Can you work these out from the model? Positions are in its coordinate system, mm. Face numbers are marked on the shaded views. A direction names the side the tool comes from. Coordinates: 2 decimals unless noted, no trailing zeros. Order: outer loops, then holes, each group sorted by start corner. A loop starts at its lowest first (then second) coordinate and runs counter-clockwise, first axis right, second up. Notation, with made-up numbers: (20.5, 68) -> (67.5, 68) arc R16 ccw to (67.5, 83) -> close; hole circle Ø9 at (9, -23). An arc over 180 degrees is marked (long way). Return JSON: item names as keys, results as strings. Group by question number.
1) If we section it at C-C, the plane y = 11: Please give me the cut outline in (x, z) (3 decimals).
2) Thinking about a two-plate mould opening in Y: for the marked faces 3, 4 and 5, which applies, +Y half, -Y half, draft (parallel to the pull), parting line (faces both ways), or undercut?
3) For the marked faces 1 and 2, which set-ups out of +Z, -Z, +X, -X, +Y, -Y let a thin tool reach every point of the face, with its end or its side?
4) For pin 1 (3 mm diameter, centred on x = 8.5, y = 8.5, fed in from -Z); pin 2 (1 mm diameter, centred on x = 4, y = 11.5, fed in from +Z); pin 3 (10 mm diameter, centred on x = -10, z = 3, fed in from -Y); pin 4 (3 mm diameter, centred on y = 2.5, z = 7.5, fed in from +X), each with a flat end and sliding along its axis, tell me the tip position at first contact or that it passes through.
5) If I drill on probe 1 along Z at (x, y) = (0, 9.5) (3 decimals); probe 2 along Z at (x, y) = (0, 3.75); probe 3 along Y at (x, z) = (7.5, 7.5), over which ranges is the centre line in solid material (lowest first)? Write a range as from..to.
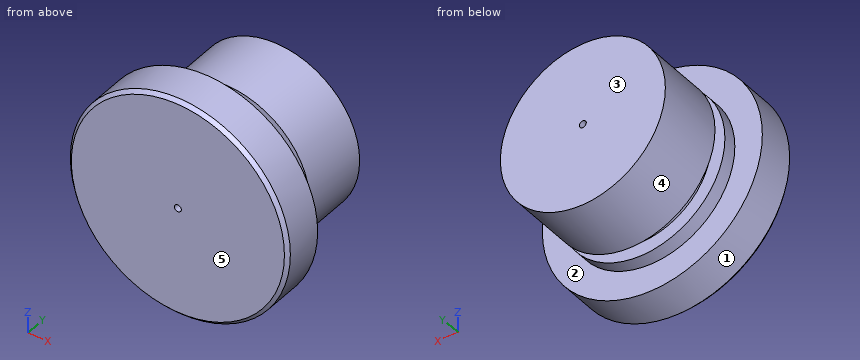
from build123d import *

# Parameters (mm, degrees)
SKETCH1_R           = 12.7
BOSS_EXTRUDE1_DEPTH = 15.875
SKETCH2_R           = 12.7
SKETCH2_R_2         = 9.525
CUT_EXTRUDE1_DEPTH  = 11.1125
SKETCH3_R           = 0.396875
CUT_EXTRUDE2_DEPTH  = 16.875
CHAMFER1_SIZE       = 0.396875
SKETCH4_R           = 9.525
SKETCH4_R_2         = 7.9375
CUT_EXTRUDE3_DEPTH  = 1.5875


with BuildPart() as part:
    # Sketch1 → Boss-Extrude1 (new body)
    with BuildSketch(Plane(origin=(0, 0, 0), x_dir=(1, 0, 0), z_dir=(0, 1, 0))):
        Circle(SKETCH1_R)
    extrude(amount=BOSS_EXTRUDE1_DEPTH)

    # Sketch2 → Cut-Extrude1 (cut)
    with BuildSketch(Plane(origin=(0, 15.875, 0), x_dir=(1, 0, 0), z_dir=(0, 1, 0))):
        Circle(SKETCH2_R)
        Circle(SKETCH2_R_2, mode=Mode.SUBTRACT)
    extrude(amount=-CUT_EXTRUDE1_DEPTH, mode=Mode.SUBTRACT)

    # Sketch3 → Cut-Extrude2 (cut, through all)
    with BuildSketch(Plane.XZ):
        Circle(SKETCH3_R)
    extrude(amount=-CUT_EXTRUDE2_DEPTH, mode=Mode.SUBTRACT)

    # Chamfer1
    chamfer1_edges = [part.edges().sort_by_distance(p)[0] for p in [
        (-12.7, 0, 0),
    ]]
    chamfer(chamfer1_edges, length=CHAMFER1_SIZE)

    # Sketch4 → Cut-Extrude3 (cut)
    with BuildSketch(Plane(origin=(0, 6.35, 0), x_dir=(1, 0, 0), z_dir=(0, 1, 0))):
        Circle(SKETCH4_R)
        Circle(SKETCH4_R_2, mode=Mode.SUBTRACT)
    extrude(amount=CUT_EXTRUDE3_DEPTH, mode=Mode.SUBTRACT)


solid = part.part
Result sheet:
{
 "1": {"outline": "circle Ø19.05 at (0, 0); hole circle Ø0.794 at (0, 0)"},
 "2": {"face 3": "+Y half", "face 4": "draft", "face 5": "-Y half"},
 "3": {"face 1": "+Y, -Y", "face 2": "+Y"},
 "4": {"pin 1": "stops at z = -6.46", "pin 2": "stops at z = 8.86", "pin 3": "stops at y = 0", "pin 4": "stops at x = 11.19"},
 "5": {"probe 1": "z = -9.525..-0.397, 0.397..9.525", "probe 2": "z = -12.7..-0.4, 0.4..12.7", "probe 3": "y = 0..4.76"}
}
